```python
from build123d import *

# Parameters (mm, degrees)
F0_R     = 8.5
F1_DEPTH = 1.5875
F2_DEPTH = 12.7
F3_DEPTH = 6.35


with BuildPart() as f1:
    # F0 (on Front) → F1 (new body)
    with BuildSketch(Plane.XZ):
        with BuildLine():
            Line((4.92, 50.64), (-45.56, 50.64))
            ThreePointArc((-45.56, 50.64), (-49.1521024484, 49.1521024484), (-50.64, 45.56))
            Line((-50.64, 45.56), (-50.64, -4.92))
            ThreePointArc((-50.64, -4.92), (-49.1521024484, -8.5121024484), (-45.56, -10))
            Line((-45.56, -10), (4.92, -10))
            ThreePointArc((4.92, -10), (8.5121024484, -8.5121024484), (10, -4.92))
            Line((10, -4.92), (10, 45.56))
            ThreePointArc((10, 45.56), (8.5121024484, 49.1521024484), (4.92, 50.64))
        make_face()
        with BuildLine():
            ThreePointArc((-49.624, 44.544), (-48.1361024484, 48.1361024484), (-44.544, 49.624))
            Line((-44.544, 49.624), (3.904, 49.624))
            ThreePointArc((3.904, 49.624), (7.4961024484, 48.1361024484), (8.984, 44.544))
            Line((8.984, 44.544), (8.984, -3.904))
            ThreePointArc((8.984, -3.904), (7.4961024484, -7.4961024484), (3.904, -8.984))
            Line((3.904, -8.984), (-44.544, -8.984))
            ThreePointArc((-44.544, -8.984), (-48.1361024484, -7.4961024484), (-49.624, -3.904))
            Line((-49.624, -3.904), (-49.624, 44.544))
        make_face(mode=Mode.SUBTRACT)
        with BuildLine():
            Line((3.904, 49.624), (-44.544, 49.624))
            ThreePointArc((-44.544, 49.624), (-48.1361024484, 48.1361024484), (-49.624, 44.544))
            Line((-49.624, 44.544), (-49.624, -3.904))
            ThreePointArc((-49.624, -3.904), (-48.1361024484, -7.4961024484), (-44.544, -8.984))
            Line((-44.544, -8.984), (3.904, -8.984))
            ThreePointArc((3.904, -8.984), (7.4961024484, -7.4961024484), (8.984, -3.904))
            Line((8.984, -3.904), (8.984, 44.544))
            ThreePointArc((8.984, 44.544), (7.4961024484, 48.1361024484), (3.904, 49.624))
        make_face()
        with BuildLine():
            ThreePointArc((-40.64, 35.56), (-39.1521024484, 39.1521024484), (-35.56, 40.64))
            Line((-35.56, 40.64), (-5.08, 40.64))
            ThreePointArc((-5.08, 40.64), (-1.4878975516, 39.1521024484), (0, 35.56))
            Line((0, 35.56), (0, 5.08))
            ThreePointArc((0, 5.08), (-1.4878975516, 1.4878975516), (-5.08, 0))
            Line((-5.08, 0), (-35.56, 0))
            ThreePointArc((-35.56, 0), (-39.1521024484, 1.4878975516), (-40.64, 5.08))
            Line((-40.64, 5.08), (-40.64, 35.56))
        make_face(mode=Mode.SUBTRACT)
        with BuildLine():
            Line((-5.08, 40.64), (-35.56, 40.64))
            ThreePointArc((-35.56, 40.64), (-39.1521024484, 39.1521024484), (-40.64, 35.56))
            Line((-40.64, 35.56), (-40.64, 5.08))
            ThreePointArc((-40.64, 5.08), (-39.1521024484, 1.4878975516), (-35.56, 0))
            Line((-35.56, 0), (-5.08, 0))
            ThreePointArc((-5.08, 0), (-1.4878975516, 1.4878975516), (0, 5.08))
            Line((0, 5.08), (0, 35.56))
            ThreePointArc((0, 35.56), (-1.4878975516, 39.1521024484), (-5.08, 40.64))
        make_face()
        with Locations((-29.845, 10.795)):
            Circle(F0_R, mode=Mode.SUBTRACT)
        with Locations((-10.795, 10.795)):
            Circle(F0_R, mode=Mode.SUBTRACT)
        with Locations((-29.845, 29.845)):
            Circle(F0_R, mode=Mode.SUBTRACT)
        with Locations((-10.795, 29.845)):
            Circle(F0_R, mode=Mode.SUBTRACT)
        with Locations((-10.795, 29.845)):
            Circle(F0_R)
        with Locations((-29.845, 29.845)):
            Circle(F0_R)
        with Locations((-29.845, 10.795)):
            Circle(F0_R)
        with Locations((-10.795, 10.795)):
            Circle(F0_R)
    extrude(amount=-F1_DEPTH)

    # F0 (on Front) → F2 (join)
    with BuildSketch(Plane.XZ):
        with BuildLine():
            Line((-5.08, 40.64), (-35.56, 40.64))
            ThreePointArc((-35.56, 40.64), (-39.1521024484, 39.1521024484), (-40.64, 35.56))
            Line((-40.64, 35.56), (-40.64, 5.08))
            ThreePointArc((-40.64, 5.08), (-39.1521024484, 1.4878975516), (-35.56, 0))
            Line((-35.56, 0), (-5.08, 0))
            ThreePointArc((-5.08, 0), (-1.4878975516, 1.4878975516), (0, 5.08))
            Line((0, 5.08), (0, 35.56))
            ThreePointArc((0, 35.56), (-1.4878975516, 39.1521024484), (-5.08, 40.64))
        make_face()
        with Locations((-29.845, 10.795)):
            Circle(F0_R, mode=Mode.SUBTRACT)
        with Locations((-10.795, 10.795)):
            Circle(F0_R, mode=Mode.SUBTRACT)
        with Locations((-29.845, 29.845)):
            Circle(F0_R, mode=Mode.SUBTRACT)
        with Locations((-10.795, 29.845)):
            Circle(F0_R, mode=Mode.SUBTRACT)
    extrude(amount=F2_DEPTH)

    # F0 (on Front) → F3 (join)
    with BuildSketch(Plane.XZ):
        with BuildLine():
            Line((4.92, 50.64), (-45.56, 50.64))
            ThreePointArc((-45.56, 50.64), (-49.1521024484, 49.1521024484), (-50.64, 45.56))
            Line((-50.64, 45.56), (-50.64, -4.92))
            ThreePointArc((-50.64, -4.92), (-49.1521024484, -8.5121024484), (-45.56, -10))
            Line((-45.56, -10), (4.92, -10))
            ThreePointArc((4.92, -10), (8.5121024484, -8.5121024484), (10, -4.92))
            Line((10, -4.92), (10, 45.56))
            ThreePointArc((10, 45.56), (8.5121024484, 49.1521024484), (4.92, 50.64))
        make_face()
        with BuildLine():
            ThreePointArc((-49.624, 44.544), (-48.1361024484, 48.1361024484), (-44.544, 49.624))
            Line((-44.544, 49.624), (3.904, 49.624))
            ThreePointArc((3.904, 49.624), (7.4961024484, 48.1361024484), (8.984, 44.544))
            Line((8.984, 44.544), (8.984, -3.904))
            ThreePointArc((8.984, -3.904), (7.4961024484, -7.4961024484), (3.904, -8.984))
            Line((3.904, -8.984), (-44.544, -8.984))
            ThreePointArc((-44.544, -8.984), (-48.1361024484, -7.4961024484), (-49.624, -3.904))
            Line((-49.624, -3.904), (-49.624, 44.544))
        make_face(mode=Mode.SUBTRACT)
    extrude(amount=F3_DEPTH)


solid = f1.part
```
Part model, mm, in its own coordinate system. A direction names the side the tool comes from. Coordinates: 2 decimals unless noted, no trailing zeros. Write each loop counter-clockwise with the first axis right and the second up, starting at its lowest first coordinate (ties: lowest second). Pieces come first, ordered by that corner, then holes.
Item 1: Slice it at A-A (y = -1.5). Write the cut outline in (x, z) (3 decimals).
Item 2: Slice it at C-C (x = -3.5). Write the cut outline in (y, z), and give its area (3 significant figures).
Item 3: Mould opens along X. For faces 3 (the face through (-21, -2, -10)), 4 (the face through (-50.64, -2, 21)), 5 (the face through (-11.902, -6.261, 38.273)) say: released by +X, released by -X, zero draft, split by the parting line, or undercut.
Item 4: Slice it at D-D (y = -9.5). Write the cut outline in (x, z) (3 decimals), and give its area (3 significant figures).
Item 5: Probe line 1 (Z direction, x = -9, y = -2); line 2 (X direction, y = -2.75, z = -4); line 3 (Z direction, x = -27.5, y = -10.5). List the from-to ranges inside material, lowest first.
Item 6: Pin check, flat tips, straight feed: pin 1 (13.5 mm diameter, centred on x = -10.795, z = 10.795, fed in from -Y); pin 2 (4 mm diameter, centred on y = -8.5, z = 27.5, fed in from +X); pin 3 (6 mm diameter, centred on x = -11, y = -11, fed in from -Z). Stop position of each tip, or through.
Item 7: Slice it at B-B (z = -2.5). Write the cut outline in (x, y), and give its area (3 significant figures).
Item 8: Which spindle directions (+Z, -Z, +X, -X, +Y, -Y) get a long thin tool onto all of the face, cutting with end or side? Do faces 1 (the face through (-49.112, -2.326, 49.191)), 2 (the face through (-48.175, -3.131, 48.096)). Say none if no direction does.
Results found:
1. outline: (-50.64, -4.92) arc R5.08 ccw to (-45.56, -10) - (4.92, -10) arc R5.08 ccw to (10, -4.92) - (10, 45.56) arc R5.08 ccw to (4.92, 50.64) - (-45.56, 50.64) arc R5.08 ccw to (-50.64, 45.56) - close; (-40.64, 5.08) arc R5.08 ccw to (-35.56, 0) - (-5.08, 0) arc R5.08 ccw to (0, 5.08) - (0, 35.56) arc R5.08 ccw to (-5.08, 40.64) - (-35.56, 40.64) arc R5.08 ccw to (-40.64, 35.56) - close; hole (-49.624, -3.904) arc R5.08 ccw to (-44.544, -8.984) - (3.904, -8.984) arc R5.08 ccw to (8.984, -3.904) - (8.984, 44.544) arc R5.08 ccw to (3.904, 49.624) - (-44.544, 49.624) arc R5.08 ccw to (-49.624, 44.544) - close; hole circle Ø17 at (-29.845, 10.795); hole circle Ø17 at (-29.845, 29.845); hole circle Ø17 at (-10.795, 10.795); hole circle Ø17 at (-10.795, 29.845)
2. outline: (-12.7, 0.25) - (0, 0.25) - (0, -8.98) - (-6.35, -8.98) - (-6.35, -10) - (1.59, -10) - (1.59, 50.64) - (-6.35, 50.64) - (-6.35, 49.62) - (0, 49.62) - (0, 40.39) - (-12.7, 40.39) - (-12.7, 34.21) - (0, 34.21) - (0, 25.48) - (-12.7, 25.48) - (-12.7, 15.16) - (0, 15.16) - (0, 6.43) - (-12.7, 6.43) - close
2. area: 397 mm2
3. face 3: zero draft
3. face 4: released by -X
3. face 5: undercut
4. outline: (-40.64, 5.08) arc R5.08 ccw to (-35.56, 0) - (-5.08, 0) arc R5.08 ccw to (0, 5.08) - (0, 35.56) arc R5.08 ccw to (-5.08, 40.64) - (-35.56, 40.64) arc R5.08 ccw to (-40.64, 35.56) - close; hole circle Ø17 at (-29.845, 10.795); hole circle Ø17 at (-29.845, 29.845); hole circle Ø17 at (-10.795, 10.795); hole circle Ø17 at (-10.795, 29.845)
4. area: 722 mm2
5. line 1: z = -10 to -8.98, 0 to 2.49, 19.1 to 21.54, 38.15 to 40.64, 49.62 to 50.64
5. line 2: x = -50.64 to -49.62, 8.98 to 10
5. line 3: z = 0 to 2.62, 18.97 to 21.67, 38.02 to 40.64
6. pin 1: stops at y = 0
6. pin 2: stops at x = 0
6. pin 3: stops at z = 0
7. outline: (-50.64, -6.35) - (-49.62, -6.35) - (-49.62, 0) - (8.98, 0) - (8.98, -6.35) - (10, -6.35) - (10, 1.59) - (-50.64, 1.59) - close
7. area: 109 mm2
8. face 1: +Z, -X, +Y, -Y
8. face 2: -Y
